from build123d import *

# Parameters (mm, degrees)
SKETCH1_R           = 5
SKETCH1_R_2         = 25
BOSS_EXTRUDE1_DEPTH = 10


with BuildPart() as part:
    # Sketch1 → Boss-Extrude1 (new body)
    with BuildSketch(Plane.XY):
        with BuildLine():
            Line((60, 10), (38.729833462, 10))
            ThreePointArc((38.729833462, 10), (34.641016151, 20), (28.025170769, 28.541019662))
            Line((28.025170769, 28.541019662), (38.660254038, 46.961524227))
            ThreePointArc((38.660254038, 46.961524227), (35, 60.621778265), (21.339745962, 56.961524227))
            Line((21.339745962, 56.961524227), (10.704662693, 38.541019662))
            ThreePointArc((10.704662693, 38.541019662), (0, 40), (-10.704662693, 38.541019662))
            Line((-10.704662693, 38.541019662), (-21.339745962, 56.961524227))
            ThreePointArc((-21.339745962, 56.961524227), (-35, 60.621778265), (-38.660254038, 46.961524227))
            Line((-38.660254038, 46.961524227), (-28.025170769, 28.541019662))
            ThreePointArc((-28.025170769, 28.541019662), (-34.641016151, 20), (-38.729833462, 10))
            Line((-38.729833462, 10), (-60, 10))
            ThreePointArc((-60, 10), (-70, 0), (-60, -10))
            Line((-60, -10), (-38.729833462, -10))
            ThreePointArc((-38.729833462, -10), (-34.641016151, -20), (-28.025170769, -28.541019662))
            Line((-28.025170769, -28.541019662), (-38.660254038, -46.961524227))
            ThreePointArc((-38.660254038, -46.961524227), (-35, -60.621778265), (-21.339745962, -56.961524227))
            Line((-21.339745962, -56.961524227), (-10.704662693, -38.541019662))
            ThreePointArc((-10.704662693, -38.541019662), (0, -40), (10.704662693, -38.541019662))
            Line((10.704662693, -38.541019662), (21.339745962, -56.961524227))
            ThreePointArc((21.339745962, -56.961524227), (35, -60.621778265), (38.660254038, -46.961524227))
            Line((38.660254038, -46.961524227), (28.025170769, -28.541019662))
            ThreePointArc((28.025170769, -28.541019662), (34.641016151, -20), (38.729833462, -10))
            Line((38.729833462, -10), (60, -10))
            ThreePointArc((60, -10), (70, 0), (60, 10))
        make_face()
        with Locations((60, 0)):
            Circle(SKETCH1_R, mode=Mode.SUBTRACT)
        with Locations((30, -51.961524227)):
            Circle(SKETCH1_R, mode=Mode.SUBTRACT)
        with Locations((-30, -51.961524227)):
            Circle(SKETCH1_R, mode=Mode.SUBTRACT)
        with Locations((-60, 0)):
            Circle(SKETCH1_R, mode=Mode.SUBTRACT)
        with Locations((-30, 51.961524227)):
            Circle(SKETCH1_R, mode=Mode.SUBTRACT)
        with Locations((30, 51.961524227)):
            Circle(SKETCH1_R, mode=Mode.SUBTRACT)
        Circle(SKETCH1_R_2, mode=Mode.SUBTRACT)
    extrude(amount=BOSS_EXTRUDE1_DEPTH)


solid = part.part
Here's how the part is built. I have some questions about the finished solid (model axes, mm). A direction names the side the tool comes from. Give positions to 0.01 mm unless a question says otherwise; leave off trailing zeros. Order: outer loops, then holes, each group sorted by start corner. A loop starts at its lowest first (then second) coordinate and runs counter-clockwise, first axis right, second up. Notation, with made-up numbers: M 4,67 L 18,67 A26 ccw 18,98 Z; hole C 2,-6 d2. An arc over 180 degrees is marked long. Answer as a JSON object with one key per item and string values. Group by question number.
1) I'm going to push flat-ended pins straight in: pin 1 Ø6 at (x, y) = (-30, 51.96) entering from +Z; pin 2 Ø3 at (x, z) = (49.5, 3.5) entering from -Y; pin 3 Ø2 at (y, z) = (-33.5, 2.5) entering from -X; pin 4 Ø5 at (y, z) = (-46, 5) entering from -X. Where does each tip first touch, or does it pass through?
2) Suppose I cut it at C-C, the plane z = 3.25. Count the separate pieces of the cut face and the enclosed holes in it, plus the area to 3 significant figures.
3) We'd pull the mould along X, two halves only. Please class faces 1 (the flat face through (-26, 0, 10)), 2 (the flat face through (33.417, -37.88, 4.93)), 3 (the cylindrical face through (23.846, 7.509, 4.93)): pulls with the +X half, pulls with the -X half, needs draft (parallel to the pull), parting line crosses it, or undercut.
4) On a 3-axis mill with a long thin cutter (end or side, diameter ignored), from which of +Z, -Z, +X, -X, +Y, -Y can I reach the whole of each face in a straight line? I mean faces 4 (the flat face through (33.268, 37.622, 4.93)), 5 (the flat face through (16.097, 47.88, 4.93)), 6 (the cylindrical face through (-34.565, 20.131, 4.93)). Say none if no direction works.
5) Suppose I cut it at B-B, the plane y = -49.5. Write out the boundary of the cut face in (x, z), plus the area to 3 significant figures.
6) Suppose I cut it at A-A, the plane x = 0. Write out the boundary of the cut face in (y, z).
7) Suppose I cut it at D-D, the plane x = -30. Write out the boundary of the cut face in (y, z), plus the area to 3 significant figures.
8) Please list where these lines run through material, in increasing order: L1, parallel to X at y = 53.5, z = 4.75; L2, parallel to X at y = 50, z = 4; L3, parallel to Y at x = 33, z = 0.75. Write a range as [from, to].
Results found:
{
 "1": {"pin 1": "through", "pin 2": "y = -10", "pin 3": "x = -31.47", "pin 4": "x = -39.38"},
 "2": {"separate pieces": "1", "enclosed holes": "7", "area": "5,980 mm²"},
 "3": {"face 1": "needs draft", "face 2": "pulls with the +X half", "face 3": "undercut"},
 "4": {"face 4": "+Z, -Z, +X", "face 5": "+Z, -Z, +Y", "face 6": "+Z, -Z, -X"},
 "5": {"outline": "M -39.69,0 L -34.35,0 L -34.35,10 L -39.69,10 Z; M -25.65,0 L -17.03,0 L -17.03,10 L -25.65,10 Z; M 17.03,0 L 25.65,0 L 25.65,10 L 17.03,10 Z; M 34.35,0 L 39.69,0 L 39.69,10 L 34.35,10 Z", "area": "279 mm²"},
 "6": {"outline": "M -40,0 L -25,0 L -25,10 L -40,10 Z; M 25,0 L 40,0 L 40,10 L 25,10 Z"},
 "7": {"outline": "M -61.96,0 L -56.96,0 L -56.96,10 L -61.96,10 Z; M -46.96,0 L -31.96,0 L -31.96,10 L -46.96,10 Z; M -26.46,0 L 26.46,0 L 26.46,10 L -26.46,10 Z; M 31.96,0 L 46.96,0 L 46.96,10 L 31.96,10 Z; M 56.96,0 L 61.96,0 L 61.96,10 L 56.96,10 Z", "area": "929 mm²"},
 "8": {"L1": "[-39.88, -34.76], [-25.24, -19.34], [19.34, 25.24], [34.76, 39.88]", "L2": "[-39.81, -34.6], [-25.4, -17.32], [17.32, 25.4], [34.6, 39.81]", "L3": "[-61.5, -55.96], [-47.96, -37.16], [-22.61, 22.61], [37.16, 47.96], [55.96, 61.5]"}
}
